Autodesk Inventor part; units mm, degrees
ref_plane "YZ Plane" through (0, 0, 0) normal (1, 0, 0) x (0, 1, 0)
ref_plane "XZ Plane" through (0, 0, 0) normal (0, 1, 0) x (-1, 0, 0)
ref_plane "XY Plane" through (0, 0, 0) normal (0, 0, 1) x (1, 0, 0)
sketch "Эскиз1" plane through (0, 0, 0) normal (0, 0, 1) x (1, 0, 0)
  circle A0 centre (0, 0) radius 2.4
  circle A1 centre (0, 0) radius 1.75
  circle A2 centre (0, 0) radius 1.5
  circle A3 centre (0, 0) radius 2.5
  line L0 (0, 0) -> (0, 4) construction
  circle A4 centre (0, 2) radius 0.5
  dimension "d0" = 4.8
  dimension "d1" = 3.5
  dimension "d2" = 3
  dimension "d3" = 5
extrude "Выдавливание1" add sketch "Эскиз1" along normal mid plane 6.8 contours A0 A4 A1 | A4 A1 A0
extrude "Выдавливание2" add sketch "Эскиз1" along normal mid plane 5.2 contours A4 A1 A0 | A0 A4 | A1 A4 picked at (-0.2377, 2.1059) picked at (0, 1.6632)
pattern_circular "Круговой массив1" count 8 over 360 about axis through (0, 0, 0) along (0, 0, 1) of "Выдавливание2"
fillet "Сопряжение1" radius 0.2 2 edges at (-2.4, 0, 3.4) (-2.4, 0, -3.4)
properties part number "роликовый подшипник"
The listing builds one solid part. Answer for the finished solid, in the listing's coordinates (mm). A direction names the side the tool comes from. Give positions to 0.01 mm unless a question says otherwise; leave off trailing zeros. Write each loop counter-clockwise with the first axis right and the second up, starting at its lowest first coordinate (ties: lowest second). Pieces come first, ordered by that corner, then holes. Notation, with made-up numbers: (-12.75, -21.5) -> (9.25, -21.5) arc R17 ccw to (9.25, 0.5) -> close; hole circle Ø6 at (8, 34.5). An arc over 180 degrees is marked (long way). Write item = value, one per line. Start each with the question number.
1) The part is cut by section A-A, the plane x = 0. Determine the outline of the cut face in (y, z), and give its area (3 significant figures).
2) Which of the six approach directions +Z, -Z, +X, -X, +Y, -Y give full straight-line access (tool end or side, diameter ignored) to faces 1 (the face through (1.617, -0.67, 0.048)), 2 (the face through (0, -2, 3.4)), 3 (the face through (-1.5, 0, 0))?
3) Determine the mould class of faces 4 (the face through (2.217, -0.919, 0.045)), 5 (the face through (0, -2, -3.4)), 6 (the face through (0, 1.5, 0)) for opening direction X: +X half, -X half, draft (parallel to the pull), parting line (faces both ways), or undercut.
4) Each of these flat-tipped pins is pushed along its axis until it touches: pin 1 (0.6 mm diameter, centred on x = 1, y = 1, fed in from +Z); pin 2 (0.5 mm diameter, centred on x = 2, y = -1.5, fed in from -Z). Where does it stop, or does it pass through?
5) Straight lines are drawn through the part: line 1 along Y through (x, z) = (0, -1); line 2 along Z through (x, y) = (-1.7, 0). For each, find the intervals that lie inside material, in ascending order.
Solutions:
q1.outline = (-2.5, -2.6) -> (-2.4, -2.6) -> (-2.4, -3.2) arc R0.2 ccw to (-2.2, -3.4) -> (-1.75, -3.4) -> (-1.75, -2.6) -> (-1.5, -2.6) -> (-1.5, 2.6) -> (-1.75, 2.6) -> (-1.75, 3.4) -> (-2.2, 3.4) arc R0.2 ccw to (-2.4, 3.2) -> (-2.4, 2.6) -> (-2.5, 2.6) -> close; (1.5, -2.6) -> (1.75, -2.6) -> (1.75, -3.4) -> (2.2, -3.4) arc R0.2 ccw to (2.4, -3.2) -> (2.4, -2.6) -> (2.5, -2.6) -> (2.5, 2.6) -> (2.4, 2.6) -> (2.4, 3.2) arc R0.2 ccw to (2.2, 3.4) -> (1.75, 3.4) -> (1.75, 2.6) -> (1.5, 2.6) -> close
q1.area = 12.4 mm²
q2.face_1 = none
q2.face_2 = +Z, +X, -X, +Y, -Y
q2.face_3 = +Z, -Z
q3.face_4 = parting line
q3.face_5 = draft
q3.face_6 = undercut
q4.pin_1 = 2.6
q4.pin_2 = -3.39
q5.line_1 = -2.5 to -1.5, 1.5 to 2.5
q5.line_2 = -2.6 to 2.6
